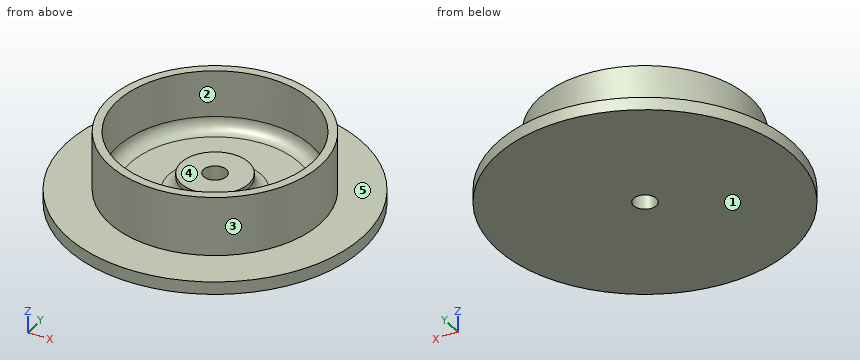
```python
from build123d import *

# Parameters (mm, degrees)
F0_R     = 35
F1_DEPTH = 3
F2_R     = 25
F2_R_2   = 23
F3_DEPTH = 14
F4_R     = 8
F5_DEPTH = 4
F6_R     = 2.7
F7_DEPTH = 25
F8_R     = 3


with BuildPart() as f1:
    # F0 (on Top) → F1 (new body)
    with BuildSketch(Plane.XY):
        Circle(F0_R)
    extrude(amount=F1_DEPTH)

    # F2 (on face) → F3 (join)
    with BuildSketch(Plane.XY.offset(3)):
        Circle(F2_R)
        Circle(F2_R_2, mode=Mode.SUBTRACT)
    extrude(amount=F3_DEPTH)

    # F4 (on face) → F5 (join)
    with BuildSketch(Plane.XY.offset(3)):
        Circle(F4_R)
    extrude(amount=F5_DEPTH)

    # F6 (on face) → F7 (cut)
    with BuildSketch(Plane.XY.offset(7)):
        Circle(F6_R)
    extrude(amount=-F7_DEPTH, mode=Mode.SUBTRACT)

    # F8
    f8_edges = [f1.edges().sort_by_distance(p)[0] for p in [
        (-23, 0, 3),
        (-8, 0, 3),
    ]]
    fillet(f8_edges, radius=F8_R)


solid = f1.part
```
Check sheet for the modelled part. Datum: model origin and axes. Units: mm. Face numbers are marked on the shaded views. A direction names the side the tool comes from. Coordinates: 2 decimals unless noted, no trailing zeros. Order: outer loops, then holes, each group sorted by start corner. A loop starts at its lowest first (then second) coordinate and runs counter-clockwise, first axis right, second up. Notation, with made-up numbers: M -32,-33 L -5,-33 A17 ccw -5,-9 Z; hole C -11.5,75 d6. An arc over 180 degrees is marked long. Write each question's results on one line, items separated by ' | '. Start each with the question number.
1. Material ranges on probe 1 along Y at (x, z) = (0, 2); probe 2 along Y at (x, z) = (0, 10.25); probe 3 along Y at (x, z) = (0, 5.25), recorded low to high.
2. Mould release check, pull along Y, two halves, no side actions. Record for the marked faces 3, 4 and 5: +Y half, -Y half, draft (parallel to the pull), parting line (faces both ways), or undercut.
3. Access from +Z, -Z, +X, -X, +Y, -Y to the whole of each face (thin tool, end or side, straight path). Record for the marked faces 1 and 2.
4. Go/stop test with flat-tipped pins: P1, Ø2, axis at x = -11, y = -27.5, coming from the +Z side; P2, Ø8, axis at x = 25, z = 10, coming from the -Y side; P3, Ø1.5, axis at x = 21.5, z = 15, coming from the +Y side. Record where each tip stops, or that it passes through.
5. Cross-section at D-D on x = -24. Record the cut outline in (y, z).
6. Cross-section at A-A on y = 0. Record the cut outline in (x, z).
7. Cross-section at C-C on z = 14. Record the cut outline in (x, y), and give its area (3 significant figures).
Checks:
1) probe 1: y = -35 to -2.7, 2.7 to 35 | probe 2: y = -25 to -23, 23 to 25 | probe 3: y = -25 to -22.9, -8.1 to -2.7, 2.7 to 8.1, 22.9 to 25
2) face 3: parting line | face 4: undercut | face 5: draft
3) face 1: -Z, +X, -X, +Y, -Y | face 2: +Z
4) P1: stops at z = 3 | P2: stops at y = -13.56 | P3: stops at y = 13.94
5) outline: M -25.48,0 L 25.48,0 L 25.48,3 L 7,3 L 7,17 L -7,17 L -7,3 L -25.48,3 Z
6) outline: M -35,0 L -2.7,0 L -2.7,7 L -8,7 L -8,6 A3 cw -11,3 L -20,3 A3 cw -23,6 L -23,17 L -25,17 L -25,3 L -35,3 Z; M 2.7,0 L 35,0 L 35,3 L 25,3 L 25,17 L 23,17 L 23,6 A3 cw 20,3 L 11,3 A3 cw 8,6 L 8,7 L 2.7,7 Z
7) outline: C 0,0 d50; hole C 0,0 d46 | area: 302 mm²
